```python
from build123d import *

# Parameters (mm, degrees)
BOSS_EXTRUDE1_DEPTH = 3
SKETCH2_W           = 3
SKETCH2_H           = 2.54
SKETCH2_H_2         = 6
BOSS_EXTRUDE2_DEPTH = 3


with BuildPart() as part:
    # Sketch1 → Boss-Extrude1 (new body)
    with BuildSketch(Plane.XY):
        Polygon((-3, 0), (-11, 0), (-11, 3), (-14, 3), (-14, 0), (-20, 0), (-20, -26.54), (0, -15), (30, -15), (30, 0), (0, 0), (0, 3), (-3, 3), align=None)
    extrude(amount=BOSS_EXTRUDE1_DEPTH)

    # Sketch2 → Boss-Extrude2 (add)
    with BuildSketch(Plane.XY.offset(3)):
        with Locations((-21.5, -1.27)):
            Rectangle(SKETCH2_W, SKETCH2_H)
        with Locations((-21.5, -11.54)):
            Rectangle(SKETCH2_W, SKETCH2_H_2)
        with Locations((-21.5, -23.54)):
            Rectangle(SKETCH2_W, SKETCH2_H_2)
    extrude(amount=-BOSS_EXTRUDE2_DEPTH)


solid = part.part
```
For this review, take the finished solid that the model builds, in its own axes (mm). A direction names the side the tool comes from. Round coordinates to 2 decimals unless told otherwise and drop trailing zeros. Write each loop counter-clockwise with the first axis right and the second up, starting at its lowest first coordinate (ties: lowest second). Pieces come first, ordered by that corner, then holes. Notation, with made-up numbers: (-38, 88) -> (-24, 88) arc R15 cw to (-24, 103) -> close; hole circle Ø8 at (49, -8.75). An arc over 180 degrees is marked (long way). One line per question, with ' | ' between items. Start each with the question number.
(1) Add section D-D, the plane x = -12. Write out the cut boundary in (y, z).
(2) Add section B-B, the plane z = 1.5. Write out the cut boundary in (x, y).
(3) Mouldability with a two-part tool opening along Y and no side actions: class faces 6 (the face through (15, -15, 1)), 7 (the face through (-22, -20.54, 2)), 8 (the face through (3, -8, 0)) as released by +Y, released by -Y, zero draft, split by the parting line, or undercut.
(4) Add section A-A, the plane y = 1. Write out the cut boundary in (x, z).
(5) Tool access review of faces 1 (the face through (-19, 0, 2)), 2 (the face through (-1, 3, 1)), 3 (the face through (30, -8, 1)), 4 (the face through (-7, 0, 1)), 5 (the face through (-22, -2.54, 2)): name each direction out of +Z, -Z, +X, -X, +Y, -Y from which nothing blocks a thin tool from reaching the whole face with its end or side.
(6) Add section C-C, the plane x = 7.5. Write out the cut boundary in (y, z), plus the area to 3 significant figures.
(7) For line 1 along X through (y, z) = (1, 0.9); line 2 along X through (y, z) = (-5.5, 2.15); line 3 along Y through (x, z) = (24.5, 2.5), list the stretches that pass through material, from the lowest coordinate up. Write a range as from..to.
(8) Insertion check: P1, Ø1.5, axis at x = -19.5, z = 1, coming from the +Y side; P2, Ø1.5, axis at y = 1.5, z = 1, coming from the +X side; P3, Ø0.9, axis at y = 2, z = 2, coming from the -X side. Each pin has a flat end and moves straight along its axis. Give the tip position at first contact, or say it passes through.
Answer list:
1) outline: (-21.92, 0) -> (3, 0) -> (3, 3) -> (-21.92, 3) -> close
2) outline: (-23, -26.54) -> (-20, -26.54) -> (0, -15) -> (30, -15) -> (30, 0) -> (0, 0) -> (0, 3) -> (-3, 3) -> (-3, 0) -> (-11, 0) -> (-11, 3) -> (-14, 3) -> (-14, 0) -> (-23, 0) -> (-23, -2.54) -> (-20, -2.54) -> (-20, -8.54) -> (-23, -8.54) -> (-23, -14.54) -> (-20, -14.54) -> (-20, -20.54) -> (-23, -20.54) -> close
3) face 6: released by -Y | face 7: undercut | face 8: zero draft
4) outline: (-14, 0) -> (-11, 0) -> (-11, 3) -> (-14, 3) -> close; (-3, 0) -> (0, 0) -> (0, 3) -> (-3, 3) -> close
5) face 1: +Z, -Z, -X, +Y | face 2: +Z, -Z, +X, -X, +Y | face 3: +Z, -Z, +X, +Y, -Y | face 4: +Z, -Z, +Y | face 5: +Z, -Z, -X
6) outline: (-15, 0) -> (0, 0) -> (0, 3) -> (-15, 3) -> close | area: 45.0 mm²
7) line 1: -14..-11, -3..0 | line 2: -20..30 | line 3: -15..0
8) P1: y = 0 | P2: x = 0 | P3: x = -14
